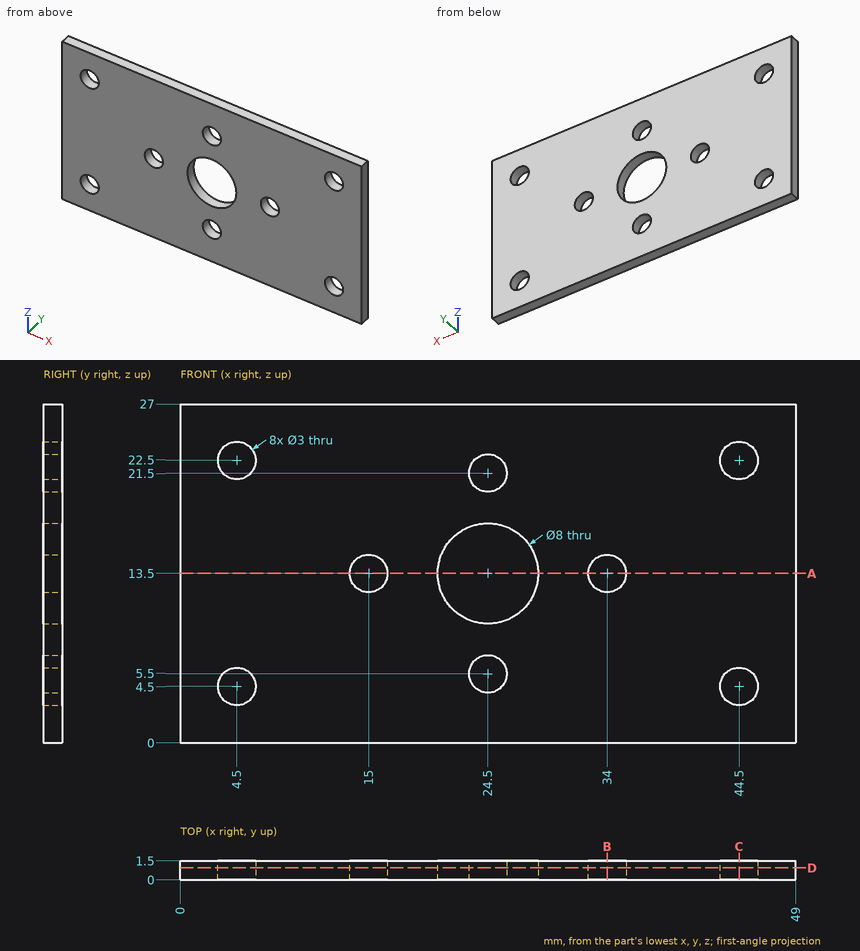
Design review of the part shown in the three views and the two pictorial views. Dimensions are in mm from the part's minimum x, y and z. Round coordinates to 2 decimals unless told otherwise and drop trailing zeros. Order: outer loops, then holes, each group sorted by start corner. A loop starts at its lowest first (then second) coordinate and runs counter-clockwise, first axis right, second up. Notation, with made-up numbers: (65, 28.5) - (106, 28.5) arc R35 cw to (106, 66.5) - close; hole circle Ø5 at (-11.5, 4). An arc over 180 degrees is marked (long way). Answer in a Markdown table with one row per item.
(1) Take a section at B-B on x = 34. Write out the cut boundary in (y, z), plus the area to 3 significant figures.
Result set:
| item | result |
|---|---|
| outline | (0, 0) - (1.5, 0) - (1.5, 12) - (0, 12) - close; (0, 15) - (1.5, 15) - (1.5, 27) - (0, 27) - close |
| area | 36.0 mm2 |
(2) Take a section at C-C on x = 44.5. Write out the cut boundary in (y, z).
Result set:
| item | result |
|---|---|
| outline | (0, 0) - (1.5, 0) - (1.5, 3) - (0, 3) - close; (0, 6) - (1.5, 6) - (1.5, 21) - (0, 21) - close; (0, 24) - (1.5, 24) - (1.5, 27) - (0, 27) - close |
(3) Take a section at D-D on y = 0.95. Count the separate pieces of the cut face and the enclosed holes in it, plus the area to 3 significant figures.
Result set:
| item | result |
|---|---|
| separate pieces | 1 |
| enclosed holes | 9 |
| area | 1,220 mm2 |
(4) Take a section at A-A on z = 13.5. Write out the cut boundary in (x, y), plus the area to 3 significant figures.
Result set:
| item | result |
|---|---|
| outline | (0, 0) - (13.5, 0) - (13.5, 1.5) - (0, 1.5) - close; (16.5, 0) - (20.5, 0) - (20.5, 1.5) - (16.5, 1.5) - close; (28.5, 0) - (32.5, 0) - (32.5, 1.5) - (28.5, 1.5) - close; (35.5, 0) - (49, 0) - (49, 1.5) - (35.5, 1.5) - close |
| area | 52.5 mm2 |
(5) For line 1 (Z direction, x = 44.5, y = 0.65); line 2 (X direction, y = 1.05, z = 13.5); line 3 (Z direction, x = 23.5, y = 1.05), list the stretches that pass through material, from the lowest coordinate up. Write a range as from..to.
Result set:
| item | result |
|---|---|
| line 1 | z = 0..3, 6..21, 24..27 |
| line 2 | x = 0..13.5, 16.5..20.5, 28.5..32.5, 35.5..49 |
| line 3 | z = 0..4.38, 6.62..9.63, 17.37..20.38, 22.62..27 |
(6) Clearance check with flat-ended pins moving along their axes: P1, Ø4, axis at x = 44.5, z = 4.5, coming from the +Y side; P2, Ø2.5, axis at x = 24.5, z = 5.5, coming from the +Y side. State where each tip first meets the part, or that it passes through.
Result set:
| item | result |
|---|---|
| P1 | stops at y = 1.5 |
| P2 | passes through |
